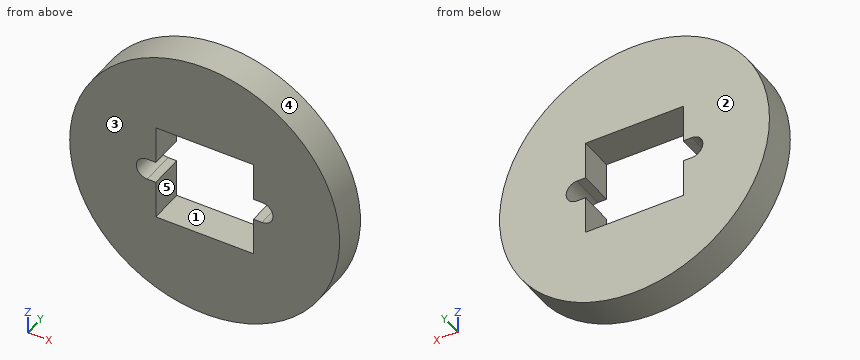
Autodesk Inventor part; units mm, degrees
ref_plane "YZ Plane" through (0, 0, 0) normal (1, 0, 0) x (0, 1, 0)
ref_plane "XZ Plane" through (0, 0, 0) normal (0, 1, 0) x (-1, 0, 0)
ref_plane "XY Plane" through (0, 0, 0) normal (0, 0, 1) x (1, 0, 0)
sketch "Эскиз1" plane through (0, 0, 0) normal (0, 1, 0) x (-1, 0, 0)
  line L0 (8.5, -8.5) -> (-8.5, -8.5)
  line L1 (-8.5, -8.5) -> (-8.5, -1.9)
  line L2 (-8.5, 8.5) -> (8.5, 8.5)
  line L3 (8.5, 8.5) -> (8.5, 1.9)
  line L4 (0, 0) -> (0, -10.3494) construction
  line L5 (0, 0) -> (-17.6402, 0) construction
  circle A0 centre (10, 0) radius 0.9 construction
  circle A1 centre (-10, 0) radius 0.9 construction
  arc A2 (10, -1.9) -> (10, 1.9) centre (10, 0) ccw
  line L6 (10, -1.9) -> (8.5, -1.9)
  line L7 (10, 1.9) -> (8.5, 1.9)
  line L8 (8.5, -1.9) -> (8.5, -8.5)
  line L9 (8.5, 1.9) -> (8.5, -1.9) construction
  circle A3 centre (-10, 0) radius 0.9 construction
  arc A4 (-10, 1.9) -> (-10, -1.9) centre (-10, 0) ccw
  line L10 (-10, -1.9) -> (-8.5, -1.9)
  line L11 (-10, 1.9) -> (-8.5, 1.9)
  line L12 (-8.5, -1.9) -> (-8.5, 1.9) construction
  line L13 (-8.5, 1.9) -> (-8.5, 8.5)
  circle A5 centre (0, 0) radius 23.5
  dimension "d0" = 17
  dimension "d1" = 17
  dimension "d2" = 1.8
  dimension "d3" = 20
  dimension "d4" = 3.8
  dimension "d5" = 47
extrude "Выдавливание1" add sketch "Эскиз1" along normal blind 6
sketch "Эскиз2" plane through (0, 0, 0) normal (0, 1, 0) x (-1, 0, 0)
  circle A0 centre (0, 0) radius 23.5 construction
  line L0 (8.5, -1.9) -> (8.5, -8.5) construction
  line L1 (8.5, -8.5) -> (-8.5, -8.5) construction
  line L2 (-8.5, -8.5) -> (-8.5, -1.9) construction
  line L3 (-8.5, -1.9) -> (-10, -1.9) construction
  arc A1 (-10, 1.9) -> (-10, -1.9) centre (-10, 0) ccw construction
  line L4 (-10, 1.9) -> (-8.5, 1.9) construction
  line L5 (-8.5, 1.9) -> (-8.5, 8.5) construction
  line L6 (-8.5, 8.5) -> (8.5, 8.5) construction
  line L7 (8.5, 8.5) -> (8.5, 1.9) construction
  line L8 (8.5, 1.9) -> (10, 1.9) construction
  arc A2 (10, -1.9) -> (10, 1.9) centre (10, 0) ccw construction
  line L9 (10, -1.9) -> (8.5, -1.9) construction
  circle A3 centre (14.713, -5.2) radius 1.4
  line L10 (0, 0) -> (0, -23.5) construction
  circle A4 centre (-14.713, -5.2) radius 1.4
  arc A5 (12.5706, -3.1) -> (16.8554, -3.1) centre (14.713, -5.2) ccw
  arc A6 (-16.8554, -3.1) -> (-12.5706, -3.1) centre (-14.713, -5.2) ccw
  line L11 (14.713, -5.2) -> (14.713, -3.1) construction
  line L12 (16.8554, -3.1) -> (12.5706, -3.1)
  line L13 (-16.8554, -3.1) -> (-12.5706, -3.1)
  dimension "d8" = 2.8
  dimension "d9" = 3.3
  dimension "d10" = 29.426
  dimension "d11" = 6
  dimension "d14" = 2.1
extrude "Выдавливание2" [suppressed]
properties part number "circle_cutout"
Verification items for the finished model (mm, model axes). Face numbers are marked on the shaded views. A direction names the side the tool comes from. Give positions to 0.01 mm unless a question says otherwise; leave off trailing zeros. Loops run counter-clockwise (first coordinate to the right, second up) from the corner with the lowest first, then second, coordinate; pieces in that order, holes last. Notation, with made-up numbers: (5.25, 32.5) - (36.25, 32.5) arc R17 ccw to (36.25, 45.5) - close; hole circle Ø3 at (67.5, 12). An arc over 180 degrees is marked (long way). Write each question's results on one line, items separated by ' | '.
1) Material ranges on L1, parallel to Z at x = -0.5, y = 0.5; L2, parallel to Z at x = -3, y = 1.65; L3, parallel to X at y = 5.45, z = 7, recorded low to high. Write a range as from..to.
Solution:
L1: -23.49..-8.5, 8.5..23.49 | L2: -23.31..-8.5, 8.5..23.31 | L3: -22.43..-8.5, 8.5..22.43
2) Mould release check, pull along Z, two halves, no side actions. Record for the marked faces 3, 4 and 5: pulls with the +Z half, pulls with the -Z half, needs draft (parallel to the pull), parting line crosses it, or undercut.
Solution:
face 3: needs draft | face 4: parting line crosses it | face 5: undercut
3) Sectioned sample at D-D on x = 18. Record the boundary of the cut face in (y, z).
Solution:
outline: (0, -15.11) - (6, -15.11) - (6, 15.11) - (0, 15.11) - close
4) Sectioned sample at A-A on x = 0. Record the boundary of the cut face in (y, z).
Solution:
outline: (0, -23.5) - (6, -23.5) - (6, -8.5) - (0, -8.5) - close; (0, 8.5) - (6, 8.5) - (6, 23.5) - (0, 23.5) - close
5) Sectioned sample at C-C on y = 2.6. Record the boundary of the cut face in (x, z), plus the area to 3 significant figures.
Solution:
outline: circle Ø47 at (0, 0); hole (-10, -1.9) - (-8.5, -1.9) - (-8.5, -8.5) - (8.5, -8.5) - (8.5, -1.9) - (10, -1.9) arc R1.9 ccw to (10, 1.9) - (8.5, 1.9) - (8.5, 8.5) - (-8.5, 8.5) - (-8.5, 1.9) - (-10, 1.9) arc R1.9 ccw to start | area: 1,420 mm2
6) Depth check by flat-ended pin: P1, Ø1, axis at y = 4, z = -13, coming from the +X side; P2, Ø1.5, axis at x = -15.5, y = 1.5, coming from the +Z side; P3, Ø1.2, axis at x = 9, y = 4.5, coming from the -Z side; P4, Ø2, axis at x = 18.5, z = 17.5, coming from the -Y side. Enter the tip coordinate at first touch or a pass-through.
Solution:
P1: x = 19.9 | P2: z = 18.29 | P3: z = -21.95 | P4: through
7) Tool access check on the marked faces 1 and 2. Record the directions out of +Z, -Z, +X, -X, +Y, -Y that give a thin tool (end or side, any length) a straight path to the whole face; none if there is none.
Solution:
face 1: +Y, -Y | face 2: +Z, -Z, +X, -X, +Y
8) Sectioned sample at B-B on z = 0. Record the boundary of the cut face in (x, y), plus the area to 3 significant figures.
Solution:
outline: (-23.5, 0) - (-11.9, 0) - (-11.9, 6) - (-23.5, 6) - close; (11.9, 0) - (23.5, 0) - (23.5, 6) - (11.9, 6) - close | area: 139 mm2
